Input: part model. Units: mm. Frame: model coordinates. Face numbers are marked on the shaded views. Round coordinates to 2 decimals unless told otherwise and drop trailing zeros. Loops run counter-clockwise (first coordinate to the right, second up) from the corner with the lowest first, then second, coordinate; pieces in that order, holes last. Notation, with made-up numbers: (62, 20) - (81, 20) arc R6 cw to (81, 27) - close; hole circle Ø7 at (47.25, -21.5). An arc over 180 degrees is marked (long way). Write each question's results on one line, items separated by ' | '.
from build123d import *

# Parameters (mm, degrees)
F0_R     = 33.5
F1_DEPTH = 3
F2_R     = 34.5
F2_R_2   = 33.5
F3_DEPTH = 100
F4_R     = 41
F5_DEPTH = 3
F6_R     = 41
F6_R_2   = 39
F7_DEPTH = 100
F8_R     = 1
F9_R     = 0.99999


# Not quite as in the source:
# - a fillet or chamfer is up to 0.001 mm smaller than in the source, because OpenCascade refuses the exact size


with BuildPart() as f1:
    # F0 (on Top) → F1 (new body)
    with BuildSketch(Plane.XY):
        Circle(F0_R)
    extrude(amount=F1_DEPTH)

    # F2 (on Top) → F3 (join)
    with BuildSketch(Plane.XY):
        Circle(F2_R)
        Circle(F2_R_2, mode=Mode.SUBTRACT)
    extrude(amount=F3_DEPTH)

    # F4 (on Top) → F5 (join)
    with BuildSketch(Plane.XY):
        Circle(F4_R)
    extrude(amount=F5_DEPTH)

    # F6 (on Top) → F7 (join)
    with BuildSketch(Plane.XY):
        Circle(F6_R)
        Circle(F6_R_2, mode=Mode.SUBTRACT)
    extrude(amount=F7_DEPTH)

    # F8
    f8_edges = [f1.edges().sort_by_distance(p)[0] for p in [
        (-41, 0, 0),
    ]]
    fillet(f8_edges, radius=F8_R)

    # F9 (radius 1 in the source; OpenCascade refuses exactly that, so slightly less here)
    f9_edges = [f1.edges().sort_by_distance(p)[0] for p in [
        (-41, 0, 100),
        (-39, 0, 100),
    ]]
    fillet(f9_edges, radius=F9_R)


solid = f1.part
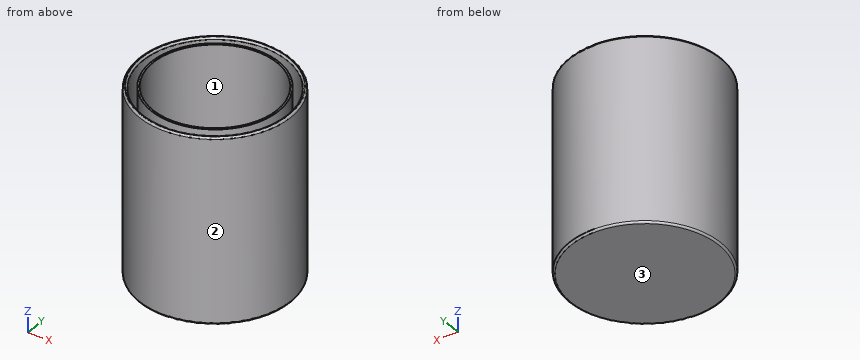
1. Section query A-A, the plane z = 87.5. Output: boundary loops of the cut face in (x, y), plus the area to 3 significant figures.
Answer:
outline: circle Ø82 at (0, 0); circle Ø69 at (0, 0); hole circle Ø78 at (0, 0); hole circle Ø67 at (0, 0) | area: 716 mm^2
2. Contact query for flat-ended pins moving along their axis: pin 1 (4 mm diameter, centred on x = 1.5, y = -12.5, fed in from +Z); pin 2 (4 mm diameter, centred on x = -8, z = 73, fed in from +Y); pin 3 (8 mm diameter, centred on y = -25, z = 86.5, fed in from +X). Output: stop coordinate, or through.
Answer:
pin 1: z = 3 | pin 2: y = 40.56 | pin 3: x = 35.21
3. Line query: line 1 (Y direction, x = 0, z = 36); line 2 (X direction, y = 8, z = 8); line 3 (X direction, y = -26, z = 59). Output: solid intervals per line, ascending. Write a range as [from, to].
Answer:
line 1: [-41, -39], [-34.5, -33.5], [33.5, 34.5], [39, 41] | line 2: [-40.21, -38.17], [-33.56, -32.53], [32.53, 33.56], [38.17, 40.21] | line 3: [-31.7, -29.07], [-22.68, -21.12], [21.12, 22.68], [29.07, 31.7]
4. Mould query, pull axis X, two halves, no side actions, for the marked faces 1, 2 and 3. Classes: pulls with the +X half, pulls with the -X half, needs draft (parallel to the pull), parting line crosses it, or undercut.
Answer:
face 1: undercut | face 2: parting line crosses it | face 3: needs draft
